Study the drawing (mm; zero at the part's minimum x, y, z) and answer. A direction names the side the tool comes from. Round coordinates to 2 decimals unless told otherwise and drop trailing zeros. Write each loop counter-clockwise with the first axis right and the second up, starting at its lowest first coordinate (ties: lowest second). Pieces come first, ordered by that corner, then holes.
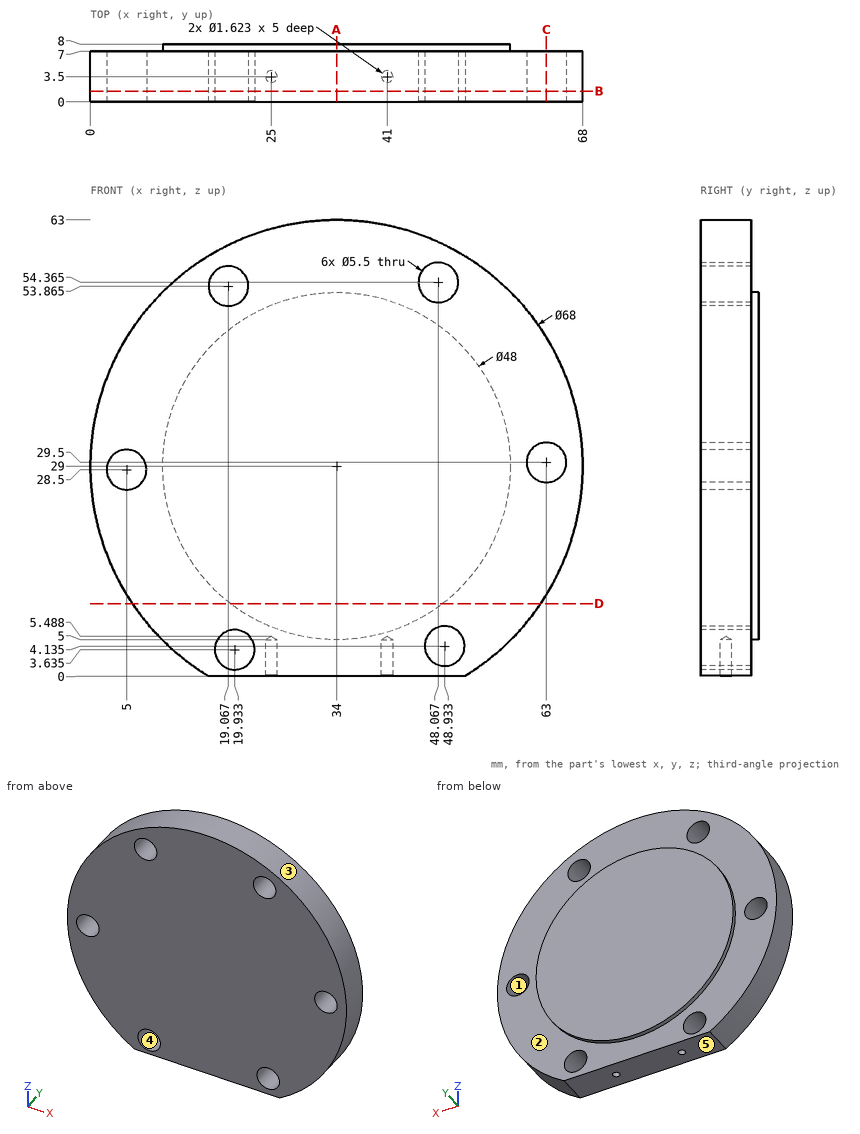
1. Straight lines are drawn through the part: line 1 along Y through (x, z) = (41, 3); line 2 along X through (y, z) = (3.25, 28) (1 decimal); line 3 along Y through (x, z) = (12, 50). For each, find the intervals that lie inside material, in ascending order.
Geometry says:
line 1: y = 0 to 2.69, 4.31 to 7
line 2: x = 0 to 2.3, 7.7 to 60.7, 65.3 to 68
line 3: y = 0 to 7
2. Section A-A on x = 34 is taken. Determine the outline of the cut face in (y, z).
Geometry says:
outline: (0, 0) - (7, 0) - (7, 5) - (8, 5) - (8, 53) - (7, 53) - (7, 63) - (0, 63) - close
3. For a pull along Z with two mould halves and no side action, classify the marked faces 3, 4 and 5 as released by +Z, released by -Z, zero draft, split by the parting line, or undercut.
Geometry says:
face 3: split by the parting line
face 4: undercut
face 5: released by -Z
4. Section D-D on z = 10 is taken. Determine the outline of the cut face in (x, y) (1 decimal), plus the area to 3 significant figures.
Geometry says:
outline: (5.8, 0) - (62.2, 0) - (62.2, 7) - (48.7, 7) - (48.7, 8) - (19.3, 8) - (19.3, 7) - (5.8, 7) - close
area: 424 mm2
5. Section B-B on y = 1.5 is taken. Give the number of separate pieces and of enclosed holes in the cut face, plus the area to 3 significant figures.
Geometry says:
separate pieces: 1
enclosed holes: 6
area: 3,370 mm2
6. Section C-C on x = 63 is taken. Determine the outline of the cut face in (y, z).
Geometry says:
outline: (0, 11.25) - (7, 11.25) - (7, 26.75) - (0, 26.75) - close; (0, 32.25) - (7, 32.25) - (7, 46.75) - (0, 46.75) - close
7. Given pin 1 (2 mm diameter, centred on x = 19.5, z = 52.5, fed in from -Y); pin 2 (4 mm diameter, centred on x = 43.5, y = 2, fed in from +Z); pin 3 (9 mm diameter, centred on x = 5, z = 28.5, fed in from +Y); pin 4 (3 mm diameter, centred on y = 5.5, z = 56, fed in from -X), each flat-ended and moving along its own axis, determine where each tip first touches the part or whether it passes through.
Geometry says:
pin 1: passes through
pin 2: stops at z = 62.16
pin 3: stops at y = 7
pin 4: stops at x = 11.51
8. A tool of negligible diameter and unlimited length cuts with its end or side. For the marked faces 1 and 2, from which of +Z, -Z, +X, -X, +Y, -Y can it reach the whole face along a straight path? Write none if from no direction.
Geometry says:
face 1: +Y, -Y
face 2: +Y
